The model under review builds one solid part; all positions refer to its coordinate system, in mm. Round coordinates to 2 decimals unless told otherwise and drop trailing zeros. Write each loop counter-clockwise with the first axis right and the second up, starting at its lowest first coordinate (ties: lowest second). Pieces come first, ordered by that corner, then holes. Notation, with made-up numbers: (63.25, -36.75) -> (91.25, -36.75) arc R12 ccw to (91.25, -23.75) -> close; hole circle Ø2 at (84.5, 36). An arc over 180 degrees is marked (long way). Answer as a JSON object with one key per item and string values. Group by question number.
1) Insertion check: pin 1 Ø8.5 at (y, z) = (0, 0) entering from +X; pin 2 Ø8 at (y, z) = (1.5, 3) entering from -X (3 decimals). Each pin has a flat end and moves straight along its axis. Give the tip position at first contact, or say it passes through.
2) We need section D-D, the plane z = -0.5. Write out the cut boundary in (x, y) (1 decimal), then the cut area to 3 significant figures.
3) We need section B-B, the plane x = 7.5. Write out the cut boundary in (y, z) (1 decimal), then the cut area to 3 significant figures.
4) Mouldability with a two-part tool opening along Z and no side actions: class faces 1 (the cylindrical face through (5.888, 4.016, -2.56)), 2 (the flat face through (-2.3, 4.4, 9.525)), 3 (the flat face through (9.525, -2.3, 4.4)) as pulls with the +Z half, pulls with the -Z half, needs draft (parallel to the pull), parting line crosses it, or undercut.
5) To check wall thickness, follow probe 1 along Y at (x, z) = (0, 7.25) (1 decimal); probe 2 along Z at (x, y) = (6.75, -0.25) (3 decimals); probe 3 along Y at (x, z) = (-4, -6.75) (3 decimals). State the ranges of each line that lie inside material, in increasing order. Write a range as [from, to].
6) We need section A-A, the plane y = 0. Write out the cut boundary in (x, z) (1 decimal), then the cut area to 3 significant figures.
from build123d import *

# Parameters (mm, degrees)
SKETCH1_W          = 19.05
SKETCH1_H          = 19.05
SKETCH1_R          = 4.7625
BASE_EXTRUDE_DEPTH = 9.525
SKETCH3_R          = 4.7625
CUT_EXTRUDE1_DEPTH = 24.3313898


with BuildPart() as part:
    # Sketch1 → Base-Extrude (new, symmetric)
    with BuildSketch(Plane.XY):
        Rectangle(SKETCH1_W, SKETCH1_H)
        with Locations(Location((0, 0, 0), (0, 0, 180))):
            Circle(SKETCH1_R, mode=Mode.SUBTRACT)
    extrude(amount=BASE_EXTRUDE_DEPTH, both=True)

    # Sketch3 → Cut-Extrude1 (cut, through all)
    with BuildSketch(Plane(origin=(9.525, 0, 0), x_dir=(0, 0, -1), z_dir=(1, 0, 0))):
        Circle(SKETCH3_R)
    extrude(amount=-CUT_EXTRUDE1_DEPTH, mode=Mode.SUBTRACT)


solid = part.part
Here are the results:
{
 "1": {"pin 1": "passes through", "pin 2": "stops at x = -9.525"},
 "2": {"outline": "(-9.5, -9.5) -> (9.5, -9.5) -> (9.5, -4.7) -> (0.5, -4.7) arc R4.8 cw to (-0.5, -4.7) -> (-9.5, -4.7) -> close; (-9.5, 4.7) -> (-0.5, 4.7) arc R4.8 cw to (0.5, 4.7) -> (9.5, 4.7) -> (9.5, 9.5) -> (-9.5, 9.5) -> close", "area": "182 mm^2"},
 "3": {"outline": "(-9.5, -9.5) -> (9.5, -9.5) -> (9.5, 9.5) -> (-9.5, 9.5) -> close; hole circle Ø9.5 at (0, 0)", "area": "292 mm^2"},
 "4": {"face 1": "undercut", "face 2": "pulls with the +Z half", "face 3": "needs draft"},
 "5": {"probe 1": "y = [-9.5, -4.8], [4.8, 9.5]", "probe 2": "z = [-9.525, -4.756], [4.756, 9.525]", "probe 3": "y = [-9.525, -2.585], [2.585, 9.525]"},
 "6": {"outline": "(-9.5, -9.5) -> (-4.8, -9.5) -> (-4.8, -4.8) -> (-9.5, -4.8) -> close; (-9.5, 4.8) -> (-4.8, 4.8) -> (-4.8, 9.5) -> (-9.5, 9.5) -> close; (4.8, -9.5) -> (9.5, -9.5) -> (9.5, -4.8) -> (4.8, -4.8) -> close; (4.8, 4.8) -> (9.5, 4.8) -> (9.5, 9.5) -> (4.8, 9.5) -> close", "area": "90.7 mm^2"}
}
